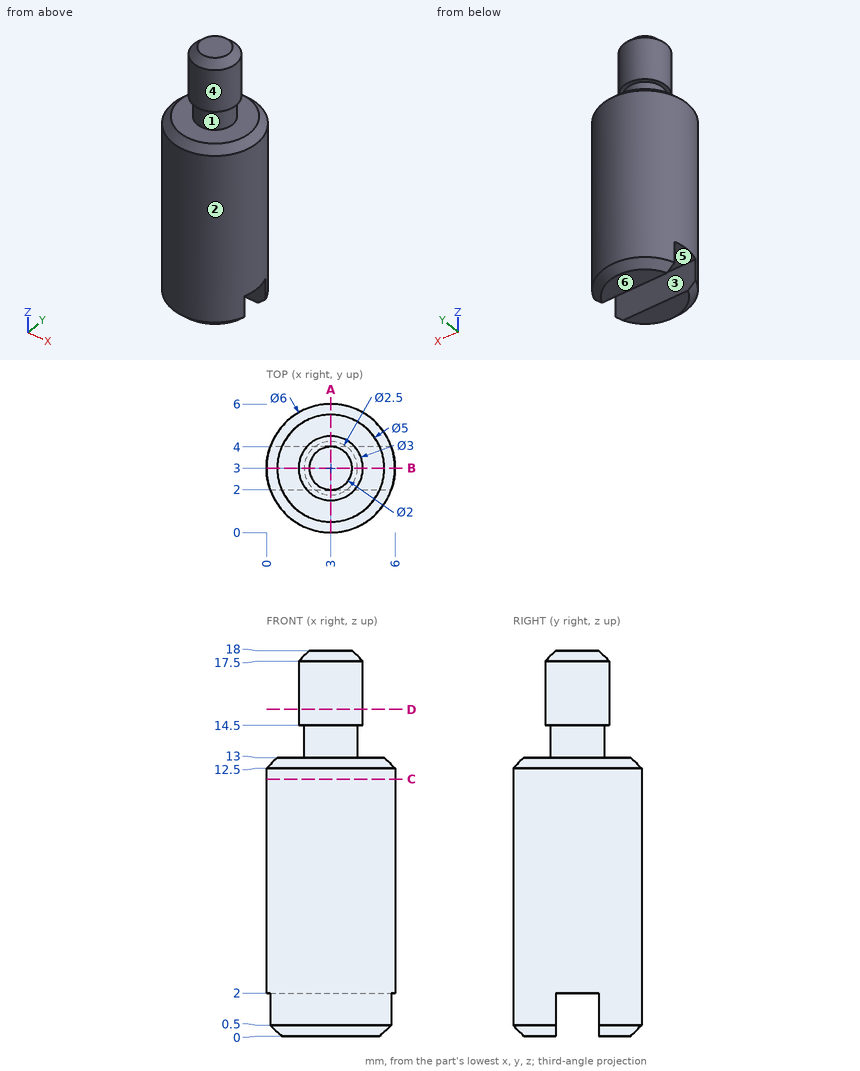
Can you work these out from the drawing? Everything is in mm from the part's minimum corner. A direction names the side the tool comes from. Round coordinates to 2 decimals unless told otherwise and drop trailing zeros. Order: outer loops, then holes, each group sorted by start corner. A loop starts at its lowest first (then second) coordinate and runs counter-clockwise, first axis right, second up. Notation, with made-up numbers: (43, 35.5) - (100, 35.5) arc R16 cw to (100, 41.5) - close; hole circle Ø3 at (28, 53). An arc over 180 degrees is marked (long way). Answer in a Markdown table with one row per item.
(1) Suppose I cut it at A-A, the plane x = 3. Please give me the cut outline in (y, z).
From the geometry:
| item | result |
|---|---|
| outline | (0, 0.5) - (0.5, 0) - (2, 0) - (2, 2) - (4, 2) - (4, 0) - (5.5, 0) - (6, 0.5) - (6, 12.5) - (5.5, 13) - (4.25, 13) - (4.25, 14.5) - (4.5, 14.5) - (4.5, 17.5) - (4, 18) - (2, 18) - (1.5, 17.5) - (1.5, 14.5) - (1.75, 14.5) - (1.75, 13) - (0.5, 13) - (0, 12.5) - close |
(2) For P1, Ø1, axis at x = 4.5, z = 1.5, coming from the -Y side; P2, Ø0.6, axis at x = 4, y = 3.5, coming from the -Z side; P3, Ø0.6, axis at x = 2, z = 1, coming from the +Y side, each with a flat end and sliding along its axis, tell me the tip position at first contact or that it passes through.
From the geometry:
| item | result |
|---|---|
| P1 | stops at y = 0.17 |
| P2 | stops at z = 2 |
| P3 | stops at y = 5.92 |
(3) Suppose I cut it at D-D, the plane z = 15.25. Please give me the cut outline in (x, y), plus the area to 3 significant figures.
From the geometry:
| item | result |
|---|---|
| outline | circle Ø3 at (3, 3) |
| area | 7.07 mm2 |
(4) If we mould it in two halves opening along Y, with no side actions, what happens to the marked faces 3, 4, 5 and 6? For each: released by +Y, released by -Y, zero draft, split by the parting line, or undercut.
From the geometry:
| item | result |
|---|---|
| face 3 | undercut |
| face 4 | split by the parting line |
| face 5 | undercut |
| face 6 | zero draft |
(5) Which directions (+Z, -Z, +X, -X, +Y, -Y) give clear straight access to the entire face, cutting with the end or side of a thin tool? Please do the marked faces 1 and 2.
From the geometry:
| item | result |
|---|---|
| face 1 | none |
| face 2 | +Z, -Z |
(6) Suppose I cut it at C-C, the plane z = 12. Please give me the cut outline in (x, y).
From the geometry:
| item | result |
|---|---|
| outline | circle Ø6 at (3, 3) |
(7) Suppose I cut it at B-B, the plane y = 3. Please give me the cut outline in (x, z).
From the geometry:
| item | result |
|---|---|
| outline | (0, 2) - (6, 2) - (6, 12.5) - (5.5, 13) - (4.25, 13) - (4.25, 14.5) - (4.5, 14.5) - (4.5, 17.5) - (4, 18) - (2, 18) - (1.5, 17.5) - (1.5, 14.5) - (1.75, 14.5) - (1.75, 13) - (0.5, 13) - (0, 12.5) - close |
(8) Please list where these lines run through material, in increasing order: L1, parallel to Z at x = 3.5, y = 0.8; L2, parallel to Y at x = 5, z = 1.5; L3, parallel to Z at x = 0.75, y = 2.25. Write a range as from..to.
From the geometry:
| item | result |
|---|---|
| L1 | z = 0..13 |
| L2 | y = 0.76..2, 4..5.24 |
| L3 | z = 2..13 |
